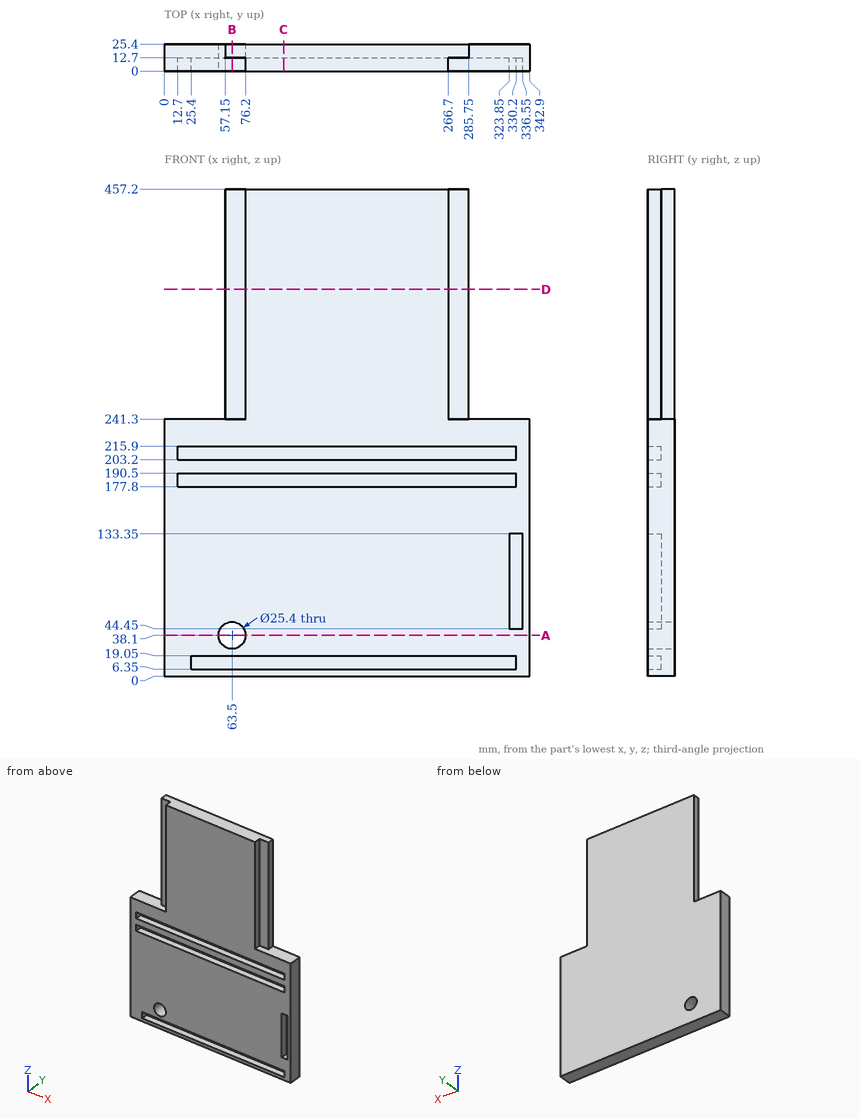
Check sheet for the drawn part. Datum: minimum x, y, z corner. Units: mm. Coordinates: 2 decimals unless noted, no trailing zeros. Loops run counter-clockwise (first coordinate to the right, second up) from the corner with the lowest first, then second, coordinate; pieces in that order, holes last. Notation, with made-up numbers: (2.25, 24) -> (20.25, 24) arc R15 ccw to (20.25, 30) -> close; hole circle Ø1 at (80, 78.25). An arc over 180 degrees is marked (long way). Write each question's results on one line, items separated by ' | '.
Item 1: Section check B-B, the plane x = 63.5. Enter the section's corners in (y, z).
Found:
outline: (0, 0) -> (25.4, 0) -> (25.4, 25.4) -> (0, 25.4) -> (0, 19.05) -> (12.7, 19.05) -> (12.7, 6.35) -> (0, 6.35) -> close; (0, 50.8) -> (25.4, 50.8) -> (25.4, 457.2) -> (12.7, 457.2) -> (12.7, 241.3) -> (0, 241.3) -> (0, 215.9) -> (12.7, 215.9) -> (12.7, 203.2) -> (0, 203.2) -> (0, 190.5) -> (12.7, 190.5) -> (12.7, 177.8) -> (0, 177.8) -> close
Item 2: Gauge pin test, flat ends, axial feed: pin 1 (8 mm diameter, centred on y = 19, z = 348.5, fed in from -X); pin 2 (4 mm diameter, centred on y = 17.5, z = 383.5, fed in from +X); pin 3 (4 mm diameter, centred on y = 9.5, z = 378.5, fed in from +X). Record the tip position at first contact, or that the pin passes through.
Found:
pin 1: stops at x = 57.15 | pin 2: stops at x = 285.75 | pin 3: stops at x = 266.7
Item 3: Section check A-A, the plane z = 38.1. Enter the section's corners in (x, y).
Found:
outline: (0, 0) -> (50.8, 0) -> (50.8, 25.4) -> (0, 25.4) -> close; (76.2, 0) -> (342.9, 0) -> (342.9, 25.4) -> (76.2, 25.4) -> close
Item 4: Section check C-C, the plane x = 112. Enter the section's corners in (y, z).
Found:
outline: (0, 0) -> (25.4, 0) -> (25.4, 457.2) -> (0, 457.2) -> (0, 215.9) -> (12.7, 215.9) -> (12.7, 203.2) -> (0, 203.2) -> (0, 190.5) -> (12.7, 190.5) -> (12.7, 177.8) -> (0, 177.8) -> (0, 19.05) -> (12.7, 19.05) -> (12.7, 6.35) -> (0, 6.35) -> close
Item 5: Section check D-D, the plane z = 363. Enter the section's corners in (x, y).
Found:
outline: (57.15, 12.7) -> (76.2, 12.7) -> (76.2, 0) -> (266.7, 0) -> (266.7, 12.7) -> (285.75, 12.7) -> (285.75, 25.4) -> (57.15, 25.4) -> close
Item 6: Material ranges on L1, parallel to Z at x = 63.5, y = 6.5; L2, parallel to Z at x = 209, y = 2; L3, parallel to X at y = 7.5, z = 65, recorded low to high.
Found:
L1: z = 0 to 6.35, 19.05 to 25.4, 50.8 to 177.8, 190.5 to 203.2, 215.9 to 241.3 | L2: z = 0 to 6.35, 19.05 to 177.8, 190.5 to 203.2, 215.9 to 457.2 | L3: x = 0 to 323.85, 336.55 to 342.9
